Geometry: final body of the model. Coordinates: model frame, mm. Face numbers are marked on the shaded views. Give positions to 0.01 mm unless a question says otherwise; leave off trailing zeros. Loops run counter-clockwise (first coordinate to the right, second up) from the corner with the lowest first, then second, coordinate; pieces in that order, holes last. Notation, with made-up numbers: M 56.5,-0.75 L 104.5,-0.75 A15 cw 104.5,26.25 Z; hole C 75,-3.5 d1. An arc over 180 degrees is marked long. Put each result on its own line as item: value.
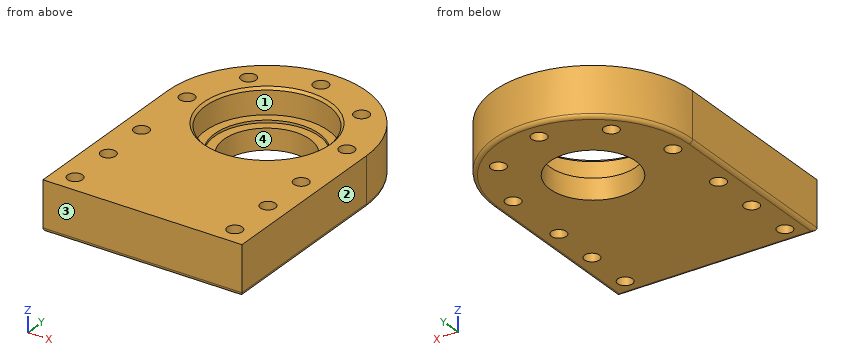
```python
from build123d import *

# Parameters (mm, degrees)
BOSS_EXTRUDE1_DEPTH = 40
SKETCH2_R           = 6.1
CUT_EXTRUDE1_DEPTH  = 40
CIRPATTERN1_COUNT   = 5
CIRPATTERN1_ANGLE   = 180
SKETCH3_R           = 6.1
CUT_EXTRUDE2_DEPTH  = 40
SKETCH4_R           = 50
CUT_EXTRUDE3_DEPTH  = 21
SKETCH5_R           = 42.5
CUT_EXTRUDE4_DEPTH  = 2
SKETCH6_R           = 35
CUT_EXTRUDE5_DEPTH  = 17
CHAMFER1_SIZE       = 2
FILLET1_R           = 3


with BuildPart() as part:
    # Sketch1 → Boss-Extrude1 (new body)
    with BuildSketch(Plane.XY):
        with BuildLine():
            Line((-81, 0), (-81, -150))
            Line((-81, -150), (81, -150))
            Line((81, -150), (81, 0))
            ThreePointArc((81, 0), (0, 81), (-81, 0))
        make_face()
    extrude(amount=BOSS_EXTRUDE1_DEPTH)

    # Sketch2 → Cut-Extrude1 (cut)
    with BuildSketch(Plane.XY.offset(40)):
        with Locations((-65, 0)):
            Circle(SKETCH2_R)
    cut_extrude1 = extrude(amount=-CUT_EXTRUDE1_DEPTH, mode=Mode.SUBTRACT)

    # CirPattern1: Cut-Extrude1 ×5 about axis
    cirpattern1_axis = Axis((0, 0, 0), (0, 0, -1))
    for i in range(1, CIRPATTERN1_COUNT):
        add(cut_extrude1.rotate(cirpattern1_axis, i * CIRPATTERN1_ANGLE / (CIRPATTERN1_COUNT - 1)), mode=Mode.SUBTRACT)

    # Sketch3 → Cut-Extrude2 (cut)
    with BuildSketch(Plane.XY.offset(40)):
        with Locations((-65, -135)):
            Circle(SKETCH3_R)
        with Locations((-65, -95)):
            Circle(SKETCH3_R)
        with Locations((-65, -55)):
            Circle(SKETCH3_R)
    cut_extrude2 = extrude(amount=-CUT_EXTRUDE2_DEPTH, mode=Mode.SUBTRACT)

    # Mirror1: Cut-Extrude2 across plane
    add(cut_extrude2.mirror(Plane(origin=(0, 0, 0), x_dir=(0, 0, 1), z_dir=(1, 0, 0))), mode=Mode.SUBTRACT)

    # Sketch4 → Cut-Extrude3 (cut)
    with BuildSketch(Plane.XY.offset(40)):
        Circle(SKETCH4_R)
    extrude(amount=-CUT_EXTRUDE3_DEPTH, mode=Mode.SUBTRACT)

    # Sketch5 → Cut-Extrude4 (cut)
    with BuildSketch(Plane.XY.offset(19)):
        Circle(SKETCH5_R)
    extrude(amount=-CUT_EXTRUDE4_DEPTH, mode=Mode.SUBTRACT)

    # Sketch6 → Cut-Extrude5 (cut)
    with BuildSketch(Plane.XY.offset(17)):
        Circle(SKETCH6_R)
    extrude(amount=-CUT_EXTRUDE5_DEPTH, mode=Mode.SUBTRACT)

    # Chamfer1
    chamfer1_edges = [part.edges().sort_by_distance(p)[0] for p in [
        (-50, 0, 40),
    ]]
    chamfer(chamfer1_edges, length=CHAMFER1_SIZE)

    # Fillet1
    fillet1_edges = [part.edges().sort_by_distance(p)[0] for p in [
        (81, -75, 0),
        (0, -150, 0),
        (-81, -75, 0),
        (0, 81, 0),
    ]]
    fillet(fillet1_edges, radius=FILLET1_R)


solid = part.part
```
Item 1: Mould query, pull axis Y, two halves, no side actions, for the marked faces 1, 2, 3 and 4. Classes: pulls with the +Y half, pulls with the -Y half, needs draft (parallel to the pull), parting line crosses it, or undercut.
Output values:
face 1: undercut
face 2: needs draft
face 3: pulls with the -Y half
face 4: undercut
Item 2: Section A-A on y = -95. Output: boundary loops of the cut face in (x, z).
Output values:
outline: M -81,3 A3 ccw -78,0 L -71.1,0 L -71.1,40 L -81,40 Z; M -58.9,0 L 58.9,0 L 58.9,40 L -58.9,40 Z; M 71.1,0 L 78,0 A3 ccw 81,3 L 81,40 L 71.1,40 Z
Item 3: Line query: probe 1 along Y at (x, z) = (-0.5, 5.5); probe 2 along Y at (x, z) = (-63, 22); probe 3 along X at (y, z) = (42.5, 16.5). Output: solid intervals per line, ascending. Write a range as [from, to].
Output values:
probe 1: [-150, -35], [35, 58.92], [71.08, 81]
probe 2: [-150, -140.76], [-129.24, -100.76], [-89.24, -60.76], [-49.24, -5.76], [5.76, 50.91]
probe 3: [-68.95, -50.98], [-40.94, 40.94], [50.98, 68.95]
Item 4: Section B-B on z = 10. Count the separate pieces of the cut face and the enclosed holes in it, then the cut area to 3 significant figures.
Output values:
separate pieces: 1
enclosed holes: 12
area: 29,500 mm²
Item 5: Pin query (flat end, axial travel): pin 1 Ø6 at (y, z) = (27.5, 6.5) entering from -X; pin 2 Ø10 at (x, y) = (65, -135) entering from -Z; pin 3 Ø4 at (x, z) = (46, 9) entering from +Y. Return the tip coordinate at first contact, or that it passes through.
Output values:
pin 1: x = -77.21
pin 2: through
pin 3: y = 68.01
